The listing builds one solid part. Answer for the finished solid, in the listing's coordinates (mm). Round coordinates to 2 decimals unless told otherwise and drop trailing zeros. Write each loop counter-clockwise with the first axis right and the second up, starting at its lowest first coordinate (ties: lowest second). Pieces come first, ordered by that corner, then holes. Notation, with made-up numbers: (-33, -16.5) - (18, -16.5) arc R27 cw to (18, 17.5) - close; hole circle Ø2 at (22.25, -13.5). An arc over 180 degrees is marked (long way). Answer as CSV lines item,"result". Start each with the question number.
Item 1: A cutting plane is placed at A-A on x = -49.5. Determine the outline of the cut face in (y, z).
Item 2: Straight lines are drawn through the part: line 1 along Z through (x, y) = (54, 1.25); line 2 along Z through (x, y) = (-104.5, 2.05); line 3 along X through (y, z) = (0.65, 10). For each, find the intervals that lie inside material, in ascending order. Write a range as [from, to].
Item 3: A cutting plane is placed at B-B on z = 58.5. Determine the outline of the cut face in (x, y), and give its area (3 significant figures).
Item 4: A cutting plane is placed at C-C on x = -11. Determine the outline of the cut face in (y, z).
Item 5: For a pull along Z with two mould halves and no side action, classify faces 1 (the flat face through (83.85, 2.03, 62.95)), 2 (the flat face through (0, 4, 7)), 3 (the flat face through (24.48, 2.03, -77.06)) as pulls with the +Z half, pulls with the -Z half, needs draft (parallel to the pull), parting line crosses it, or undercut.
Item 6: A flat-ended cylindrical pin translates along its axis: pin 1 (3 mm diameter, centred on x = 66.575, z = 49, fed in from -Y). Find the tip coordinate at first contact, or state that the pin passes through.
Item 7: A cutting plane is placed at D-D on z = 11. Determine the outline of the cut face in (x, y).
```python
from build123d import *

# Parameters (mm, degrees)
SKETCH_1_W          = 214
SKETCH_1_H          = 214
EXTRUDE_1_DEPTH     = 4
FILLET_1_R          = 3
SKETCH_2_R          = 1.6
SKETCH_2_R_2        = 1.8
CUT_EXTRUDE_1_DEPTH = 152.373709739
CUT_EXTRUDE_2_DEPTH = 152.373709739
FILLET_2_R          = 10
FILLET_3_R          = 6
FILLET_4_R          = 3
FILLET_5_R          = 6


with BuildPart() as part:
    # 스케치1 → 보스-돌출1 (new body)
    with BuildSketch(Plane(origin=(0, 0, 0), x_dir=(1, 0, 0), z_dir=(0, 1, 0))):
        Rectangle(SKETCH_1_W, SKETCH_1_H)
    extrude(amount=EXTRUDE_1_DEPTH)

    # 필렛1
    fillet_1_edges = [part.edges().sort_by_distance(p)[0] for p in [
        (107, 2, 107),
        (-107, 2, 107),
        (-107, 2, -107),
        (107, 2, -107),
    ]]
    fillet(fillet_1_edges, radius=FILLET_1_R)

    # 스케치2 → 컷-돌출1 (cut, through all)
    with BuildSketch(Plane(origin=(0, 4, 0), x_dir=(1, 0, 0), z_dir=(0, 1, 0))):
        with Locations(Location((-104.5, 104.5, 0), (0, 0, 270))):
            Circle(SKETCH_2_R)
        with Locations(Location((104.5, -104.5, 0), (0, 0, 90))):
            Circle(SKETCH_2_R)
        with Locations(Location((-104.5, -104.5, 0), (0, 0, 270))):
            Circle(SKETCH_2_R)
        with Locations(Location((104.5, 104.5, 0), (0, 0, 90))):
            Circle(SKETCH_2_R)
        with Locations(Location((-66.575, 49, 0), (0, 0, 270))):
            Circle(SKETCH_2_R_2)
        with Locations(Location((66.575, 49, 0), (0, 0, 270))):
            Circle(SKETCH_2_R_2)
        with Locations(Location((-66.575, -49, 0), (0, 0, 270))):
            Circle(SKETCH_2_R_2)
        with Locations(Location((66.575, -49, 0), (0, 0, 270))):
            Circle(SKETCH_2_R_2)
        with Locations(Location((-33.425, 49, 0), (0, 0, 270))):
            Circle(SKETCH_2_R_2)
        with Locations(Location((33.425, 49, 0), (0, 0, 90))):
            Circle(SKETCH_2_R_2)
        with Locations(Location((-33.425, -49, 0), (0, 0, 270))):
            Circle(SKETCH_2_R_2)
        with Locations(Location((33.425, -49, 0), (0, 0, 90))):
            Circle(SKETCH_2_R_2)
    extrude(amount=-CUT_EXTRUDE_1_DEPTH, mode=Mode.SUBTRACT)

    # 스케치3 → 컷-돌출2 (cut, through all)
    with BuildSketch(Plane(origin=(0, 4, 0), x_dir=(1, 0, 0), z_dir=(0, 1, 0))):
        Polygon((-97, 98), (-12, 98), (-33.5, 61.920227273), (-75.5, 61.920227273), align=None)
        Polygon((97, 98), (12, 98), (33.5, 61.920227273), (75.5, 61.920227273), align=None)
        Polygon((-97, 85.124359856), (-97, 12.875640144), (-75.575, 49), align=None)
        Polygon((97, 85.124359856), (97, 12.875640144), (75.575, 49), align=None)
        Polygon((97, -85.124359856), (97, -12.875640144), (75.575, -49), align=None)
        Polygon((-75.5, -61.920227273), (-97, -98), (-12, -98), (-33.5, -61.920227273), align=None)
        Polygon((-97, -12.875640144), (-75.575, -49), (-97, -85.124359856), align=None)
        Polygon((75.5, -61.920227273), (97, -98), (12, -98), (33.5, -61.920227273), align=None)
        Polygon((-12, 0), (-33.5, 36.079772727), (-75.5, 36.079772727), (-97, 0), (-75.5, -36.079772727), (-33.5, -36.079772727), align=None)
        Polygon((75.5, 36.079772727), (97, 0), (75.5, -36.079772727), (33.5, -36.079772727), (12, 0), (33.5, 36.079772727), align=None)
        Polygon((0, 87), (-23.035714286, 48.34310065), (0, 9.6862013), (23.035714286, 48.34310065), align=None)
        Polygon((-23.035714286, -48.34310065), (0, -9.6862013), (23.035714286, -48.34310065), (0, -87), align=None)
    extrude(amount=-CUT_EXTRUDE_2_DEPTH, mode=Mode.SUBTRACT)

    # 필렛2
    fillet_2_edges = [part.edges().sort_by_distance(p)[0] for p in [
        (-12, 2, 0),
        (-33.5, 2, 36.079772727),
        (-75.5, 2, 36.079772727),
        (-97, 2, 0),
        (-75.5, 2, -36.079772727),
        (-33.5, 2, -36.079772727),
        (33.5, 2, -36.079772727),
        (75.5, 2, -36.079772727),
        (97, 2, 0),
        (75.5, 2, 36.079772727),
        (33.5, 2, 36.079772727),
        (12, 2, 0),
    ]]
    fillet(fillet_2_edges, radius=FILLET_2_R)

    # 필렛3
    fillet_3_edges = [part.edges().sort_by_distance(p)[0] for p in [
        (97, 2, -98),
        (75.5, 2, -61.920227273),
        (33.5, 2, -61.920227273),
        (12, 2, -98),
        (-75.5, 2, 61.920227273),
        (-33.5, 2, 61.920227273),
        (-12, 2, 98),
        (-97, 2, 98),
        (33.5, 2, 61.920227273),
        (75.5, 2, 61.920227273),
        (97, 2, 98),
        (12, 2, 98),
        (-75.5, 2, -61.920227273),
        (-97, 2, -98),
        (-12, 2, -98),
        (-33.5, 2, -61.920227273),
    ]]
    fillet(fillet_3_edges, radius=FILLET_3_R)

    # 필렛4
    fillet_4_edges = [part.edges().sort_by_distance(p)[0] for p in [
        (-97, 2, -85.124359856),
        (-75.575, 2, -49),
        (-97, 2, -12.875640144),
        (75.575, 2, -49),
        (97, 2, -85.124359856),
        (97, 2, -12.875640144),
        (97, 2, 85.124359856),
        (75.575, 2, 49),
        (97, 2, 12.875640144),
        (-97, 2, 85.124359856),
        (-97, 2, 12.875640144),
        (-75.575, 2, 49),
    ]]
    fillet(fillet_4_edges, radius=FILLET_4_R)

    # 필렛5
    fillet_5_edges = [part.edges().sort_by_distance(p)[0] for p in [
        (0, 2, -87),
        (23.035714286, 2, -48.34310065),
        (0, 2, -9.6862013),
        (-23.035714286, 2, -48.34310065),
        (0, 2, 87),
        (-23.035714286, 2, 48.34310065),
        (0, 2, 9.6862013),
        (23.035714286, 2, 48.34310065),
    ]]
    fillet(fillet_5_edges, radius=FILLET_5_R)


solid = part.part
```
Geometry says:
1,outline,"(0, -107) - (4, -107) - (4, -98) - (0, -98) - close; (0, -61.92) - (4, -61.92) - (4, -36.08) - (0, -36.08) - close; (0, 36.08) - (4, 36.08) - (4, 61.92) - (0, 61.92) - close; (0, 98) - (4, 98) - (4, 107) - (0, 107) - close"
2,line 1,"z = [-107, -98], [-61.92, -36.08], [36.08, 61.92], [98, 107]"
2,line 2,"z = [-106.96, -106.1], [-102.9, 102.9], [106.1, 106.96]"
2,line 3,"x = [-107, -91.04], [-17.96, 17.96], [91.04, 107]"
3,outline,"(-107, 0) - (-97, 0) - (-97, 4) - (-107, 4) - close; (-81.21, 0) - (-16.98, 0) - (-16.98, 4) - (-81.21, 4) - close; (16.98, 0) - (81.21, 0) - (81.21, 4) - (16.98, 4) - close; (97, 0) - (107, 0) - (107, 4) - (97, 4) - close"
3,area,"594 mm^2"
4,outline,"(0, -107) - (4, -107) - (4, -68.54) - (0, -68.54) - close; (0, -28.15) - (4, -28.15) - (4, 28.15) - (0, 28.15) - close; (0, 68.54) - (4, 68.54) - (4, 107) - (0, 107) - close"
5,face 1,"undercut"
5,face 2,"needs draft"
5,face 3,"undercut"
6,pin 1,"passes through"
7,outline,"(-107, 0) - (-90.45, 0) - (-90.45, 4) - (-107, 4) - close; (-18.55, 0) - (18.55, 0) - (18.55, 4) - (-18.55, 4) - close; (90.45, 0) - (107, 0) - (107, 4) - (90.45, 4) - close"
